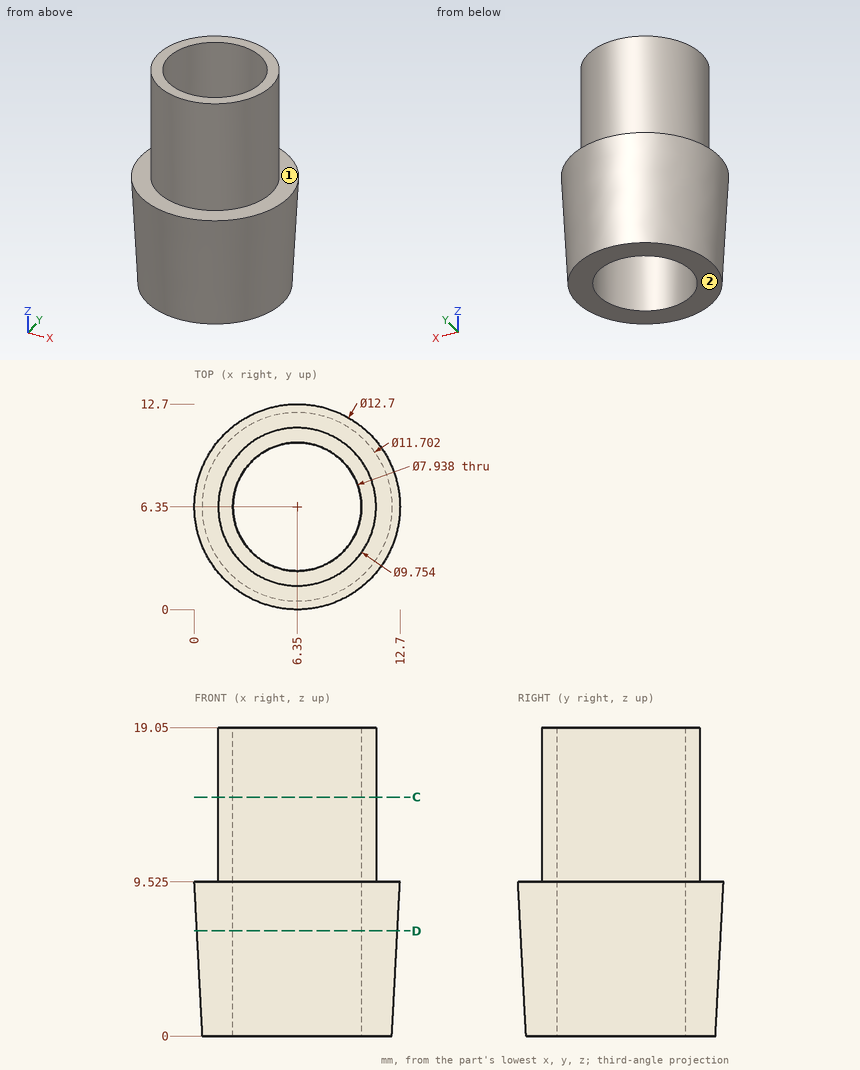
Print and shaded views of the part. All mm, measured from the part's lowest x, y and z. A direction names the side the tool comes from. Round coordinates to 2 decimals unless told otherwise and drop trailing zeros. Write each loop counter-clockwise with the first axis right and the second up, starting at its lowest first coordinate (ties: lowest second). Pieces come first, ordered by that corner, then holes. Notation, with made-up numbers: (65, -19.5) - (70, -19.5) arc R26 cw to (70, 13.5) - close; hole circle Ø3 at (85, -20). An arc over 180 degrees is marked (long way). Use CSV: the item, a comma, the result in double quotes. Start each with the question number.
Item 1: Drill centre lines: L1, parallel to Y at x = 6.35, z = 13.75; L2, parallel to Y at x = 6.35, z = 4.5; L3, parallel to Z at x = 5.25, y = 1.5 (1 decimal). Where is each one in solid material? Low to high. Write a range as [from, to].
Item 2: Band-saw the part on C-C (z = 14.75). Write the cut outline in (x, y).
Item 3: Band-saw the part on D-D (z = 6.5). Write the cut outline in (x, y).
Item 4: Pin check, flat tips, straight feed: P1, Ø1, axis at x = 6, z = 3, coming from the +Y side; P2, Ø2, axis at y = 6.5, z = 8, coming from the +X side; P3, Ø4, axis at y = 8, z = 7.5, coming from the -X side. Stop position of each tip, or through.
Item 5: Tool access for the marked faces 1 and 2: list every direction of +Z, -Z, +X, -X, +Y, -Y with a clear straight run to the whole face (end or side of a thin tool).
Checked values:
1,L1,"y = [1.47, 2.38], [10.32, 11.23]"
1,L2,"y = [0.26, 2.38], [10.32, 12.44]"
1,L3,"z = [0, 9.5]"
2,outline,"circle Ø9.75 at (6.35, 6.35); hole circle Ø7.94 at (6.35, 6.35)"
3,outline,"circle Ø12.38 at (6.35, 6.35); hole circle Ø7.94 at (6.35, 6.35)"
4,P1,"stops at y = 12.38"
4,P2,"stops at x = 12.67"
4,P3,"stops at x = 0.04"
5,face 1,"+Z"
5,face 2,"-Z, +X, -X, +Y, -Y"
